Geometry: final body of the model. Coordinates: model frame, mm. A direction names the side the tool comes from. Coordinates: 2 decimals unless noted, no trailing zeros. Loops run counter-clockwise (first coordinate to the right, second up) from the corner with the lowest first, then second, coordinate; pieces in that order, holes last. Notation, with made-up numbers: (22.25, 33) - (32.25, 33) arc R28 cw to (32.25, 61) - close; hole circle Ø8 at (33, 8.5). An arc over 180 degrees is marked (long way). Put each result on its own line as item: value. Start each with the question number.
1) Section D-D on y = 1.5. Output: boundary loops of the cut face in (x, z), and give its area (3 significant figures).
2) Section A-A on x = -11.5. Output: boundary loops of the cut face in (y, z), and give its area (3 significant figures).
3) Contact query for flat-ended pins moving along their axis: pin 1 Ø20 at (x, y) = (43.5, -16) entering from +Z; pin 2 Ø1 at (x, z) = (37.5, 4) entering from -Y; pin 3 Ø0.6 at (y, z) = (24.5, 4.5) entering from +X. Output: stop coordinate, or through.
4) Section B-B on y = 38. Output: boundary loops of the cut face in (x, z).
5) Material intervals for line 1 along Z through (x, y) = (-30.5, -25); line 2 along Y through (x, z) = (1, 2.35); line 3 along X through (y, z) = (-25, 1.55), sorted ascending. Write a range as from..to.
6) Section C-C on z = 2.1. Output: boundary loops of the cut face in (x, y).
7) Reachability of faces 1 (the flat face through (24.65, 12.675, 3.986)), 2 (the flat face through (-12.675, 24.65, 3.986)), 3 (the flat face through (0, 0, 5)), 4 (the flat face through (12.675, -24.65, 3.986)), 5 (the flat face through (-24.65, -12.675, 3.986)) from +Z, -Z, +X, -X, +Y, -Y: full face, straight path, thin tool, end or side. Return the list, or none.
```python
from build123d import *

# Parameters (mm, degrees)
F0_R          = 50
F0_R_2        = 15
F1_DEPTH      = 3
F2_DEPTH      = 5
F4_DEPTH      = 50
F5_COUNT      = 4
F6_R          = 62.5
F6_R_2        = 50
F7_DEPTH      = 25
F8_W          = 200
F8_H          = 2
F9_DEPTH      = 100
F9_DEPTH_BACK = 100


with BuildPart() as f1:
    # F0 (on Top) → F1 (new body)
    with BuildSketch(Plane.XY):
        Circle(F0_R)
        Circle(F0_R_2, mode=Mode.SUBTRACT)
    extrude(amount=F1_DEPTH)

    # F0 (on Top) → F2 (join)
    with BuildSketch(Plane.XY):
        Circle(F0_R_2)
    extrude(amount=F2_DEPTH)

    # F3 (on Front) → F4 (join)
    with BuildSketch(Plane.XZ):
        Polygon((0, 5), (0, 3), (25, 3), align=None)
    extrude(amount=F4_DEPTH)

    # F5: F1 ×4 about axis
    f5_axis = Axis((0, 0, 3), (0, 0, 1))


with BuildPart() as f1_1:
    add(f1.part)
    for i in range(1, F5_COUNT):
        add(f1.part.rotate(f5_axis, i * 360 / F5_COUNT))

    # F6 (on Top) → F7 (cut)
    with BuildSketch(Plane.XY):
        Circle(F6_R)
        Circle(F6_R_2, mode=Mode.SUBTRACT)
    extrude(amount=F7_DEPTH, mode=Mode.SUBTRACT)

    # F8 (on Front) → F9 (cut, two sides)
    with BuildSketch(Plane.XZ) as f9_sk:
        Rectangle(F8_W, F8_H)
    extrude(amount=-F9_DEPTH, mode=Mode.SUBTRACT)
    extrude(f9_sk.sketch, amount=F9_DEPTH_BACK, mode=Mode.SUBTRACT)


solid = f1_1.part
```
Answer block:
1. outline: (-49.98, 1) - (49.98, 1) - (49.98, 4.88) - (14.92, 4.88) - (14.92, 5) - (-14.92, 5) - (-14.92, 3.81) - (-25, 3) - (-49.98, 3) - close
1. area: 330 mm²
2. outline: (-48.66, 1) - (48.66, 1) - (48.66, 4.08) - (9.63, 4.08) - (9.63, 5) - (-9.63, 5) - (-9.63, 4.23) - (-25, 3) - (-48.66, 3) - close
2. area: 285 mm²
3. pin 1: stops at z = 3
3. pin 2: stops at y = 0
3. pin 3: stops at x = 0
4. outline: (-32.5, 1) - (32.5, 1) - (32.5, 3) - (0, 3) - (0, 5) - (-25, 3) - (-32.5, 3) - close
5. line 1: z = 1..3
5. line 2: y = -49.99..49.99
5. line 3: x = -43.3..43.3
6. outline: circle Ø100 at (0, 0)
7. face 1: +Z, +X, +Y
7. face 2: +Z, -X, +Y
7. face 3: +Z, +X, -X, +Y, -Y
7. face 4: +Z, +X, -Y
7. face 5: +Z, -X, -Y
